Answer from the drawing. Dimensions are ordinates in mm from the lowest x, y and z of the part. A direction names the side the tool comes from. Coordinates: 2 decimals unless noted, no trailing zeros. Order: outer loops, then holes, each group sorted by start corner. A loop starts at its lowest first (then second) coordinate and runs counter-clockwise, first axis right, second up. Notation, with made-up numbers: (70.25, -8.75) - (79.25, -8.75) arc R24 cw to (79.25, 24.25) - close; hole circle Ø1 at (61, 16.5). An arc over 180 degrees is marked (long way). Use a Markdown table: item, result. Add a question column.
Item 1: The part is cut by section D-D, the plane y = 23.5. Give the vertices of the cut face in (x, z), then the cut area to 3 significant figures.
Item 2: For the marked faces 1 and 2, determine the directions among +Z, -Z, +X, -X, +Y, -Y from which every point of the face is accessible in a straight line to the end or side of a thin tool.
Item 3: The part is cut by section C-C, the plane y = 16.5. Give the vertices of the cut face in (x, z).
Item 4: The part is cut by section B-B, the plane z = 23.75. Give the vertices of the cut face in (x, y) (3 decimals), then the cut area to 3 significant figures.
Item 5: The part is cut by section A-A, the plane y = 11. Give the vertices of the cut face in (x, z), then the cut area to 3 significant figures.
Item 6: Find the intervals of material crossed by line 1 along Z through (x, y) = (3, 26); line 2 along Y through (x, z) = (14, 11.5) (3 decimals); line 3 along Z through (x, y) = (6, 16), in increasing order.
Item 7: Flat-ended cylindrical pins translate along their axes: P1, Ø4.5, axis at x = 52.852, z = 3.298, coming from the -Y side; P2, Ø5.5, axis at x = 53, y = 9.5, coming from the -Z side. Find the tip coordinate at first contact, or state that the pin passes through.
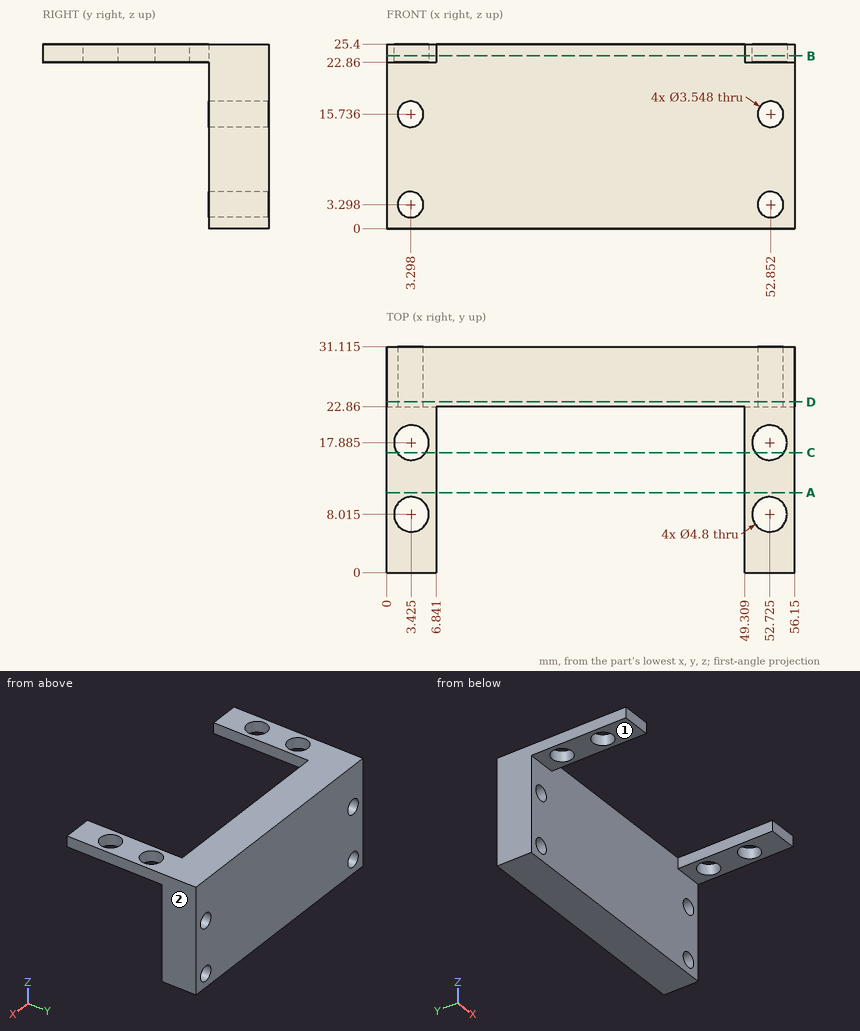
Solution:
| question | item | result |
|---|---|---|
| 1 | outline | (0, 0) - (56.15, 0) - (56.15, 25.4) - (0, 25.4) - close; hole circle Ø3.55 at (3.3, 3.3); hole circle Ø3.55 at (3.3, 15.74); hole circle Ø3.55 at (52.85, 3.3); hole circle Ø3.55 at (52.85, 15.74) |
| 1 | area | 1,390 mm2 |
| 2 | face 1 | -Z, +X, -X, -Y |
| 2 | face 2 | +Z, -Z, +X, +Y, -Y |
| 3 | outline | (0, 22.86) - (1.46, 22.86) - (1.46, 25.4) - (0, 25.4) - close; (5.39, 22.86) - (6.84, 22.86) - (6.84, 25.4) - (5.39, 25.4) - close; (49.31, 22.86) - (50.76, 22.86) - (50.76, 25.4) - (49.31, 25.4) - close; (54.69, 22.86) - (56.15, 22.86) - (56.15, 25.4) - (54.69, 25.4) - close |
| 4 | outline | (0, 0) - (6.841, 0) - (6.841, 22.86) - (49.309, 22.86) - (49.309, 0) - (56.15, 0) - (56.15, 31.115) - (0, 31.115) - close; hole circle Ø4.8 at (3.425, 8.015); hole circle Ø4.8 at (3.425, 17.885); hole circle Ø4.8 at (52.725, 8.015); hole circle Ø4.8 at (52.725, 17.885) |
| 4 | area | 704 mm2 |
| 5 | outline | (0, 22.86) - (6.84, 22.86) - (6.84, 25.4) - (0, 25.4) - close; (49.31, 22.86) - (56.15, 22.86) - (56.15, 25.4) - (49.31, 25.4) - close |
| 5 | area | 34.8 mm2 |
| 6 | line 1 | z = 0 to 1.55, 5.05 to 13.99, 17.48 to 25.4 |
| 6 | line 2 | y = 22.86 to 31.115 |
| 6 | line 3 | z = 22.86 to 25.4 |
| 7 | P1 | stops at y = 22.86 |
| 7 | P2 | stops at z = 22.86 |
